The listing builds one solid part. Answer for the finished solid, in the listing's coordinates (mm). Face numbers are marked on the shaded views. Coordinates: 2 decimals unless noted, no trailing zeros. Write each loop counter-clockwise with the first axis right and the second up, starting at its lowest first coordinate (ties: lowest second). Pieces come first, ordered by that corner, then holes.
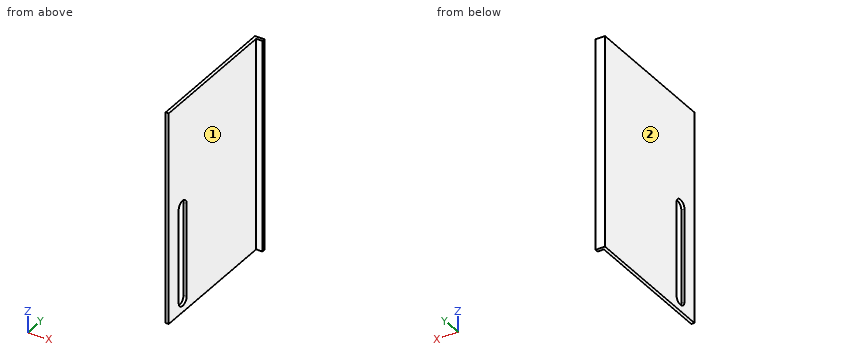
from build123d import *

# Parameters (mm, degrees)
SKETCH1_W           = 431.8
SKETCH1_H           = 285.75
BOSS_EXTRUDE1_DEPTH = 6.35
SKETCH2_W           = 431.8
SKETCH2_H           = 6.35
BOSS_EXTRUDE2_DEPTH = 12.7
CUT_EXTRUDE1_DEPTH  = 20.05


with BuildPart() as part:
    # Sketch1 → Boss-Extrude1 (new body)
    with BuildSketch(Plane(origin=(0, 0, 0), x_dir=(0, 0, -1), z_dir=(1, 0, 0))):
        Rectangle(SKETCH1_W, SKETCH1_H)
    extrude(amount=BOSS_EXTRUDE1_DEPTH)

    # Sketch2 → Boss-Extrude2 (add)
    with BuildSketch(Plane(origin=(6.35, 0, 0), x_dir=(0, 0, -1), z_dir=(1, 0, 0))):
        with Locations((0, 139.7)):
            Rectangle(SKETCH2_W, SKETCH2_H)
    extrude(amount=BOSS_EXTRUDE2_DEPTH)

    # Sketch3 → Cut-Extrude1 (cut, through all)
    with BuildSketch(Plane.ZY):
        with BuildLine():
            Line((-190.5, -85.725), (0, -85.725))
            ThreePointArc((0, -85.725), (12.7, -98.425), (0, -111.125))
            Line((0, -111.125), (-190.5, -111.125))
            ThreePointArc((-190.5, -111.125), (-203.2, -98.425), (-190.5, -85.725))
        make_face()
    extrude(amount=-CUT_EXTRUDE1_DEPTH, mode=Mode.SUBTRACT)


solid = part.part
1. Section B-B on z = 138 is taken. Give the vertices of the cut face in (x, y) (3 decimals).
Results found:
outline: (0, -142.875) - (6.35, -142.875) - (6.35, 136.525) - (19.05, 136.525) - (19.05, 142.875) - (0, 142.875) - close
2. Section D-D on y = -35.5 is taken. Give the vertices of the cut face in (x, z).
Results found:
outline: (0, -215.9) - (6.35, -215.9) - (6.35, 215.9) - (0, 215.9) - close
3. Section C-C on x = 15.25 is taken. Give the vertices of the cut face in (y, z) (3 decimals), then the cut area to 3 significant figures.
Results found:
outline: (136.525, -215.9) - (142.875, -215.9) - (142.875, 215.9) - (136.525, 215.9) - close
area: 2,740 mm2
4. Find the intervals of material crossed by L1, parallel to Y at x = 3.5, z = 0.5 (3 decimals); L2, parallel to X at y = -15.5, z = 86; L3, parallel to Y at x = 12.25, z = -23.5 (3 decimals), in increasing order.
Results found:
L1: y = -142.875 to -111.115, -85.735 to 142.875
L2: x = 0 to 6.35
L3: y = 136.525 to 142.875
5. Section A-A on z = -38 is taken. Give the vertices of the cut face in (x, y) (3 decimals), then the cut area to 3 significant figures.
Results found:
outline: (0, -142.875) - (6.35, -142.875) - (6.35, -111.125) - (0, -111.125) - close; (0, -85.725) - (6.35, -85.725) - (6.35, 136.525) - (19.05, 136.525) - (19.05, 142.875) - (0, 142.875) - close
area: 1,730 mm2
6. For a pull along X with two mould halves and no side action, classify the marked faces 1 and 2 as pulls with the +X half, pulls with the -X half, needs draft (parallel to the pull), parting line crosses it, or undercut.
Results found:
face 1: pulls with the +X half
face 2: pulls with the -X half
7. Flat-ended cylindrical pins translate along their axes: P1, Ø2, axis at x = 8.5, y = 65.5, coming from the -Z side; P2, Ø5, axis at y = -13, z = -168, coming from the +X side; P3, Ø1, axis at x = 9.5, z = 94.5, coming from the -Y side (3 decimals). Find the tip coordinate at first contact, or state that the pin passes through.
Results found:
P1: passes through
P2: stops at x = 6.35
P3: stops at y = 136.525
